For this review, take the finished solid that the model builds, in its own axes (mm). Face numbers are marked on the shaded views. Round coordinates to 2 decimals unless told otherwise and drop trailing zeros. Order: outer loops, then holes, each group sorted by start corner. A loop starts at its lowest first (then second) coordinate and runs counter-clockwise, first axis right, second up. Notation, with made-up numbers: M 67,57 L 107,57 A11 cw 107,77 Z; hole C 36.5,-18.75 d9. An arc over 180 degrees is marked long. Answer in a Markdown table with one row per item. Add a question column.
```python
from build123d import *

# Parameters (mm, degrees)
SKETCH1_R           = 98.425
SKETCH1_R_2         = 47.625
BOSS_EXTRUDE1_DEPTH = 19.05
SKETCH2_R           = 3.175
CUT_EXTRUDE1_DEPTH  = 19.05


with BuildPart() as part:
    # Sketch1 → Boss-Extrude1 (new body)
    with BuildSketch(Plane(origin=(0, 0, 0), x_dir=(1, 0, 0), z_dir=(0, 1, 0))):
        with Locations(Location((0, 0, 0), (0, 0, 90))):
            Circle(SKETCH1_R)
        with Locations(Location((0, 0, 0), (0, 0, 90))):
            Circle(SKETCH1_R_2, mode=Mode.SUBTRACT)
    extrude(amount=BOSS_EXTRUDE1_DEPTH)

    # Sketch2 → Cut-Extrude1 (cut)
    with BuildSketch(Plane(origin=(0, 19.05, 0), x_dir=(1, 0, 0), z_dir=(0, 1, 0))):
        with Locations(Location((53.362572273, 14.298458147, 0), (0, 0, 270))):
            Circle(SKETCH2_R)
        with Locations(Location((86.081449469, 23.065454869, 0), (0, 0, 270))):
            Circle(SKETCH2_R)
        with Locations(Location((40.352894367, -38.718786502, 0), (0, 0, 270))):
            Circle(SKETCH2_R)
        with Locations(Location((64.304774841, -62.670666976, 0), (0, 0, 270))):
            Circle(SKETCH2_R)
        with Locations(Location((-12.066225291, -53.960697264, 0), (0, 0, 270))):
            Circle(SKETCH2_R)
        with Locations(Location((-20.833222013, -86.67957446, 0), (0, 0, 270))):
            Circle(SKETCH2_R)
        with Locations(Location((-51.475667042, -16.185363378, 0), (0, 0, 270))):
            Circle(SKETCH2_R)
        with Locations(Location((-84.194544238, -24.9523601, 0), (0, 0, 270))):
            Circle(SKETCH2_R)
        with Locations(Location((-38.465989136, 36.831881271, 0), (0, 0, 270))):
            Circle(SKETCH2_R)
        with Locations(Location((-62.41786961, 60.783761745, 0), (0, 0, 270))):
            Circle(SKETCH2_R)
        with Locations(Location((13.953130522, 52.073792033, 0), (0, 0, 270))):
            Circle(SKETCH2_R)
        with Locations(Location((22.720127244, 84.792669229, 0), (0, 0, 270))):
            Circle(SKETCH2_R)
    extrude(amount=-CUT_EXTRUDE1_DEPTH, mode=Mode.SUBTRACT)


solid = part.part
```
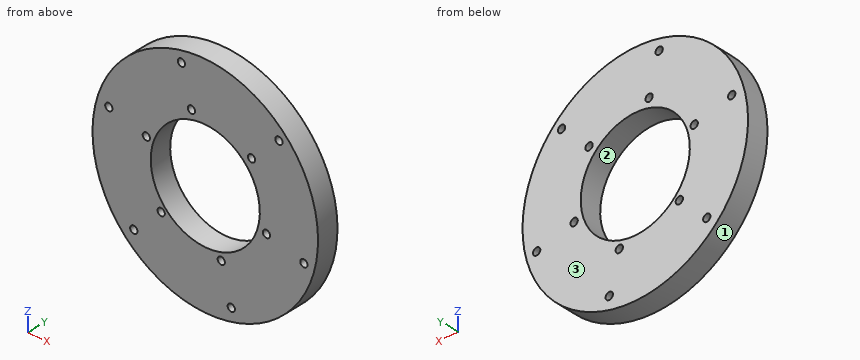
1. Consider section B-B on z = 0. Write out the cut boundary in (x, y) (3 decimals), plus the area to 3 significant figures.
2. Clearance check with flat-ended pins moving along their axes: pin 1 Ø2 at (y, z) = (2.5, 35) entering from -X; pin 2 Ø1 at (x, y) = (-76, 14) entering from +Z; pin 3 Ø6 at (x, y) = (-31, 11) entering from +Z. State where each tip first meets the part, or that it passes through.
3. Consider section C-C on y = 3.25. State how many separate pieces and enclosed holes the cut face has, plus the area to 3 significant figures.
4. To check wall thickness, follow probe 1 along X at (y, z) = (1, -22.5); probe 2 along X at (y, z) = (6, 36.5); probe 3 along X at (y, z) = (14.5, -30.5). State the ranges of each line that lie inside material, in increasing order. Write a range as [from, to].
5. The part is to be moulded in two halves that separate along Z. For the marked faces 1, 2 and 3, say which applies: pulls with the +Z half, pulls with the -Z half, needs draft (parallel to the pull), parting line crosses it, or undercut.
6. Consider section A-A on x = 0. Write out the cut boundary in (y, z) (3 decimals).
7. Consider section D-D on x = -73. Write out the cut boundary in (y, z), plus the area to 3 significant figures.
Solved:
| question | item | result |
|---|---|---|
| 1 | outline | M -98.425,0 L -47.625,0 L -47.625,19.05 L -98.425,19.05 Z; M 47.625,0 L 98.425,0 L 98.425,19.05 L 47.625,19.05 Z |
| 1 | area | 1,940 mm^2 |
| 2 | pin 1 | stops at x = -92.37 |
| 2 | pin 2 | stops at z = 63.14 |
| 2 | pin 3 | stops at z = 94.36 |
| 3 | separate pieces | 1 |
| 3 | enclosed holes | 13 |
| 3 | area | 22,900 mm^2 |
| 4 | probe 1 | x = [-95.82, -41.97], [41.97, 82.96], [89.21, 95.82] |
| 4 | probe 2 | x = [-91.41, -30.59], [30.59, 38.08], [42.62, 91.41] |
| 4 | probe 3 | x = [-93.58, -36.58], [36.58, 93.58] |
| 5 | face 1 | parting line crosses it |
| 5 | face 2 | undercut |
| 5 | face 3 | needs draft |
| 6 | outline | M 0,-98.425 L 19.05,-98.425 L 19.05,-47.625 L 0,-47.625 Z; M 0,47.625 L 19.05,47.625 L 19.05,98.425 L 0,98.425 Z |
| 7 | outline | M 0,-66.02 L 19.05,-66.02 L 19.05,66.02 L 0,66.02 Z |
| 7 | area | 2,520 mm^2 |
